Read the model definition and answer for the solid it produces. Units are mm, in the model's axes. Face numbers are marked on the shaded views. Give positions to 0.01 mm unless a question says otherwise; leave off trailing zeros. Write each loop counter-clockwise with the first axis right and the second up, starting at its lowest first coordinate (ties: lowest second). Pieces come first, ordered by that corner, then holes. Notation, with made-up numbers: M 73,-32 L 119,-32 A15 cw 119,-4 Z; hole C -1,53.5 d1. An arc over 180 degrees is marked long. Use a Markdown table: item, result. Add a question column.
Item 1: The mould has two halves that part along X. Classify the marked faces 1, 2 and 3: pulls with the +X half, pulls with the -X half, needs draft (parallel to the pull), parting line crosses it, or undercut.
Item 2: A cutting plane is placed at B-B on x = -90.5. Determine the outline of the cut face in (y, z).
Item 3: Consider probe 1 along X at (y, z) = (29, -75); probe 2 along Z at (x, y) = (-46, 34); probe 3 along Y at (x, z) = (-102.5, -78). Determine where each line is inside the solid, lowest interval first. Write a range as [from, to].
Item 4: Given P1, Ø3.5, axis at x = -75, z = -75, coming from the +Y side; P2, Ø2.5, axis at x = -104, z = -73.5, coming from the -Y side, each flat-ended and moving along its own axis, determine where each tip first touches the part or whether it passes through.
Item 5: A cutting plane is placed at A-A on z = -64.5. Determine the outline of the cut face in (x, y).
Autodesk Inventor part; units mm, degrees
ref_plane "YZ Plane" through (0, 0, 0) normal (1, 0, 0) x (0, 1, 0)
ref_plane "XZ Plane" through (0, 0, 0) normal (0, 1, 0) x (-1, 0, 0)
ref_plane "XY Plane" through (0, 0, 0) normal (0, 0, 1) x (1, 0, 0)
sketch "Sketch1" plane through (0, 0, 0) normal (0, 1, 0) x (-1, 0, 0)
  line L0 (0, 0) -> (150, 0)
  line L1 (150, 0) -> (150, -150)
  line L2 (150, -150) -> (0, -150)
  line L3 (0, -150) -> (0, 0)
  dimension "d0" = 150
  dimension "d1" = 150
extrude "Extrusion1" add sketch "Sketch1" along normal blind 50
sketch "Sketch2" plane through (0, 50, 0) normal (0, 1, 0) x (1, 0, 0)
  line L0 (-150, 150) -> (-150, 0)
  line L1 (-150, 0) -> (0, 0)
  line L2 (-133, 104) -> (-17, 104)
  line L3 (-17, 104) -> (-17, 46)
  line L4 (-17, 46) -> (-133, 46)
  line L5 (-133, 46) -> (-133, 104)
extrude "Extrusion2" cut sketch "Sketch2" against normal blind 5
sketch "Sketch3" plane through (0, 45, 0) normal (0, 1, 0) x (1, 0, 0)
  line L0 (-17, 104) -> (-17, 46)
  line L1 (-133, 46) -> (-133, 104)
  circle A0 centre (-104, 75) radius 1.5
  circle A1 centre (-75, 75) radius 1.5
  circle A2 centre (-46, 75) radius 1.5
  point P0 (0, 0)
  dimension "d14" = 3
extrude "Extrusion3" cut sketch "Sketch3" against normal up to surface (45 mm away)
sketch "Sketch4" plane through (0, 0, 0) normal (0, -1, 0) x (1, 0, 0)
  circle A0 centre (-46, -75) radius 1.5
  circle A1 centre (-46, -75) radius 4
  circle A2 centre (-75, -75) radius 1.5
  circle A3 centre (-75, -75) radius 4
  circle A4 centre (-104, -75) radius 1.5
  circle A5 centre (-104, -75) radius 4
  point P0 (0, 0)
  dimension "d17" = 8
extrude "Extrusion4" cut sketch "Sketch4" against normal blind 25 contours A0 | A1 | A2 | A3 | A4 | A5
properties part number "Base_Mount"
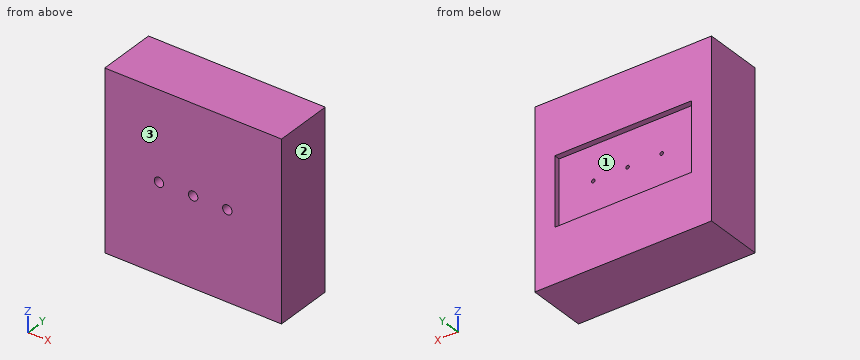
Filled in:
| question | item | result |
|---|---|---|
| 1 | face 1 | undercut |
| 1 | face 2 | pulls with the +X half |
| 1 | face 3 | needs draft |
| 2 | outline | M 0,-150 L 50,-150 L 50,-104 L 45,-104 L 45,-46 L 50,-46 L 50,0 L 0,0 Z |
| 3 | probe 1 | [-150, -105.5], [-102.5, -76.5], [-73.5, -47.5], [-44.5, 0] |
| 3 | probe 2 | [-150, -76.5], [-73.5, 0] |
| 3 | probe 3 | [25, 45] |
| 4 | P1 | y = 45 |
| 4 | P2 | y = 25 |
| 5 | outline | M -150,0 L 0,0 L 0,50 L -17,50 L -17,45 L -133,45 L -133,50 L -150,50 Z |
